Read the model definition and answer for the solid it produces. Units are mm, in the model's axes. A direction names the side the tool comes from. Round coordinates to 2 decimals unless told otherwise and drop trailing zeros. Order: outer loops, then holes, each group sorted by start corner. A loop starts at its lowest first (then second) coordinate and runs counter-clockwise, first axis right, second up.
from build123d import *

# Parameters (mm, degrees)
SKETCH1_R           = 1.5
BOSS_EXTRUDE1_DEPTH = 3


with BuildPart() as part:
    # Sketch1 → Boss-Extrude1 (new body)
    with BuildSketch(Plane(origin=(0, 0, 0), x_dir=(1, 0, 0), z_dir=(0, 1, 0))):
        Polygon((10.55, -25.469953083), (25.469953083, -10.55), (25.469953083, 10.55), (10.55, 25.469953083), (-10.55, 25.469953083), (-25.469953083, 10.55), (-25.469953083, -10.55), (-10.55, -25.469953083), align=None)
        with Locations((-17.78, 5.978)):
            Circle(SKETCH1_R, mode=Mode.SUBTRACT)
        with Locations((-17.78, -5.978)):
            Circle(SKETCH1_R, mode=Mode.SUBTRACT)
        with Locations((5.978, 17.78)):
            Circle(SKETCH1_R, mode=Mode.SUBTRACT)
        with Locations((-5.978, 17.78)):
            Circle(SKETCH1_R, mode=Mode.SUBTRACT)
        with Locations((17.78, -5.978)):
            Circle(SKETCH1_R, mode=Mode.SUBTRACT)
        with Locations((17.78, 5.978)):
            Circle(SKETCH1_R, mode=Mode.SUBTRACT)
        with Locations((-5.978, -17.78)):
            Circle(SKETCH1_R, mode=Mode.SUBTRACT)
        with Locations((5.978, -17.78)):
            Circle(SKETCH1_R, mode=Mode.SUBTRACT)
        with BuildLine():
            Line((-6.7, 23.969953083), (6.8, 23.969953083))
            ThreePointArc((6.8, 23.969953083), (8.3, 22.469953083), (6.8, 20.969953083))
            Line((6.8, 20.969953083), (-6.7, 20.969953083))
            ThreePointArc((-6.7, 20.969953083), (-8.2, 22.469953083), (-6.7, 23.969953083))
        make_face(mode=Mode.SUBTRACT)
        with BuildLine():
            Line((10.125735931, 19.550966799), (19.671677477, 10.005025253))
            ThreePointArc((19.671677477, 10.005025253), (21.792997821, 10.005025253), (21.792997821, 12.126345597))
            Line((21.792997821, 12.126345597), (12.247056275, 21.672287143))
            ThreePointArc((12.247056275, 21.672287143), (10.125735931, 21.672287143), (10.125735931, 19.550966799))
        make_face(mode=Mode.SUBTRACT)
        with BuildLine():
            Line((21.019953083, 6.65), (21.019953083, -6.85))
            ThreePointArc((21.019953083, -6.85), (22.519953083, -8.35), (24.019953083, -6.85))
            Line((24.019953083, -6.85), (24.019953083, 6.65))
            ThreePointArc((24.019953083, 6.65), (22.519953083, 8.15), (21.019953083, 6.65))
        make_face(mode=Mode.SUBTRACT)
        with BuildLine():
            Line((19.600966799, -10.175735931), (10.055025253, -19.721677477))
            ThreePointArc((10.055025253, -19.721677477), (10.055025253, -21.842997821), (12.176345597, -21.842997821))
            Line((12.176345597, -21.842997821), (21.722287143, -12.297056275))
            ThreePointArc((21.722287143, -12.297056275), (21.722287143, -10.175735931), (19.600966799, -10.175735931))
        make_face(mode=Mode.SUBTRACT)
        with BuildLine():
            Line((6.7, -21.069953083), (-6.8, -21.069953083))
            ThreePointArc((-6.8, -21.069953083), (-8.3, -22.569953083), (-6.8, -24.069953083))
            Line((-6.8, -24.069953083), (6.7, -24.069953083))
            ThreePointArc((6.7, -24.069953083), (8.2, -22.569953083), (6.7, -21.069953083))
        make_face(mode=Mode.SUBTRACT)
        with BuildLine():
            Line((-10.125735931, -19.650966799), (-19.671677477, -10.105025253))
            ThreePointArc((-19.671677477, -10.105025253), (-21.792997821, -10.105025253), (-21.792997821, -12.226345597))
            Line((-21.792997821, -12.226345597), (-12.247056275, -21.772287143))
            ThreePointArc((-12.247056275, -21.772287143), (-10.125735931, -21.772287143), (-10.125735931, -19.650966799))
        make_face(mode=Mode.SUBTRACT)
        with BuildLine():
            Line((-21.019953083, -6.75), (-21.019953083, 6.75))
            ThreePointArc((-21.019953083, 6.75), (-22.519953083, 8.25), (-24.019953083, 6.75))
            Line((-24.019953083, 6.75), (-24.019953083, -6.75))
            ThreePointArc((-24.019953083, -6.75), (-22.519953083, -8.25), (-21.019953083, -6.75))
        make_face(mode=Mode.SUBTRACT)
        with BuildLine():
            Line((-19.600966799, 10.075735931), (-10.055025253, 19.621677477))
            ThreePointArc((-10.055025253, 19.621677477), (-10.055025253, 21.742997821), (-12.176345597, 21.742997821))
            Line((-12.176345597, 21.742997821), (-21.722287143, 12.197056275))
            ThreePointArc((-21.722287143, 12.197056275), (-21.722287143, 10.075735931), (-19.600966799, 10.075735931))
        make_face(mode=Mode.SUBTRACT)
    extrude(amount=BOSS_EXTRUDE1_DEPTH)


solid = part.part
Q1. For a pull along Z with two mould halves and no side action, classify faces 1 (the face through (0, 1, 25.47)), 2 (the face through (8.3, 1.5, -22.5)), 3 (the face through (-25.47, 1, 0)) as released by +Z, released by -Z, zero draft, split by the parting line, or undercut.
Outcome:
face 1: released by +Z
face 2: undercut
face 3: zero draft
Q2. A cutting plane is placed at A-A, the plane z = -3. Give the vertices of the cut face in (x, y), plus the area to 3 significant figures.
Outcome:
outline: (-25.47, 0) - (-24.02, 0) - (-24.02, 3) - (-25.47, 3) - close; (-21.02, 0) - (21.02, 0) - (21.02, 3) - (-21.02, 3) - close; (24.02, 0) - (25.47, 0) - (25.47, 3) - (24.02, 3) - close
area: 135 mm2
Q3. Straight lines are drawn through the part: probe 1 along X at (y, z) = (2.1, -3); probe 2 along Z at (x, y) = (3.5, 0.4); probe 3 along Z at (x, y) = (17.78, 2.3). For each, find the intervals that lie inside material, in ascending order.
Outcome:
probe 1: x = -25.47 to -24.02, -21.02 to 21.02, 24.02 to 25.47
probe 2: z = -25.47 to -23.97, -20.97 to 21.07, 24.07 to 25.47
probe 3: z = -18.24 to -16.14, -11.9 to -7.48, -4.48 to 4.48, 7.48 to 12, 16.24 to 18.24
Q4. A cutting plane is placed at C-C, the plane z = -17.78. Give the vertices of the cut face in (x, y).
Outcome:
outline: (-18.24, 0) - (-16.14, 0) - (-16.14, 3) - (-18.24, 3) - close; (-11.9, 0) - (-7.48, 0) - (-7.48, 3) - (-11.9, 3) - close; (-4.48, 0) - (4.48, 0) - (4.48, 3) - (-4.48, 3) - close; (7.48, 0) - (11.9, 0) - (11.9, 3) - (7.48, 3) - close; (16.14, 0) - (18.24, 0) - (18.24, 3) - (16.14, 3) - close
Q5. A cutting plane is placed at D-D, the plane x = 18. Give the vertices of the cut face in (y, z).
Outcome:
outline: (0, -18.02) - (3, -18.02) - (3, -15.92) - (0, -15.92) - close; (0, -11.68) - (3, -11.68) - (3, -7.46) - (0, -7.46) - close; (0, -4.49) - (3, -4.49) - (3, 4.49) - (0, 4.49) - close; (0, 7.46) - (3, 7.46) - (3, 11.78) - (0, 11.78) - close; (0, 16.02) - (3, 16.02) - (3, 18.02) - (0, 18.02) - close
Q6. For faces 4 (the face through (-22.49, 1.48, -8.25)), 5 (the face through (-17.91, 1.48, -18.11)), determine the directions among +Z, -Z, +X, -X, +Y, -Y from which every point of the face is accessible in a straight line to the end or side of a thin tool.
Outcome:
face 4: +Y, -Y
face 5: -Z, -X, +Y, -Y
Q7. Flat-ended cylindrical pins translate along their axes: pin 1 (2.5 mm diameter, centred on x = -17.78, z = -5.978, fed in from +Y); pin 2 (1.5 mm diameter, centred on y = 0.5, z = 12, fed in from -X). Find the tip coordinate at first contact, or state that the pin passes through.
Outcome:
pin 1: passes through
pin 2: stops at x = -24.77
Q8. A cutting plane is placed at B-B, the plane x = -3.5. Give the vertices of the cut face in (y, z), plus the area to 3 significant figures.
Outcome:
outline: (0, -25.47) - (3, -25.47) - (3, -23.97) - (0, -23.97) - close; (0, -20.97) - (3, -20.97) - (3, 21.07) - (0, 21.07) - close; (0, 24.07) - (3, 24.07) - (3, 25.47) - (0, 25.47) - close
area: 135 mm2
